Input: part model. Units: mm. Frame: model coordinates. Face numbers are marked on the shaded views. A direction names the side the tool comes from. Give positions to 0.01 mm unless a question says otherwise; leave off trailing zeros. Loops run counter-clockwise (first coordinate to the right, second up) from the corner with the lowest first, then second, coordinate; pieces in that order, holes last. Notation, with made-up numbers: M -3,19 L 43,19 A27 ccw 43,43 Z; hole C 64,27 d5. An arc over 180 degrees is marked long. Answer as a JSON object with one key per item and string values. Group by question number.
1) Section query C-C on y = 0. Return loops of the section in (x, z), plus the area to 3 significant figures.
2) Section query D-D on z = 8.5. Return loops of the section in (x, y), plus the area to 3 significant figures.
3) Section query B-B on x = 0. Return loops of the section in (y, z), plus the area to 3 significant figures.
4) Draft query along X for the marked faces 1, 2, 3 and 4. Return one class per face: +X half, -X half, draft (parallel to the pull), parting line (faces both ways), or undercut.
5) First-contact query: P1, Ø1, axis at x = -7, z = 6, coming from the -Y side; P2, Ø11, axis at x = -3.5, y = 13, coming from the +Z side; P3, Ø3.5, axis at y = 16, z = 27, coming from the -X side; P4, Ø1, axis at x = 18, y = -18, coming from the -Z side. Flat tips, straight axial feed; report the tip coordinate or a pass-through.
6) Section query A-A on z = 15. Return loops of the section in (x, y).
7) Ray query, L1, parallel to Y at x = -15, z = 6; L2, parallel to Y at x = -7, z = 8; L3, parallel to X at y = 17, z = 25.5. Return the intervals inside material, ascending.
8) Access query for the marked faces 5, 6 and 7. Directions: +Z, -Z, +X, -X, +Y, -Y. A direction counts if a zero-diameter tool reaches every point of the face in a straight line with its end or side. Return the directions, or none.
from build123d import *

# Parameters (mm, degrees)
F1_DEPTH    = 5.08
F2_SIZE     = 5.07999
F3_DEPTH    = 12.7
F4_DEPTH    = 12.7
F5_T2_ANGLE = 254.9699407606
F5_T4_ANGLE = 254.9699407606
F8_DEPTH    = 20.32
F9_DEPTH    = 20.32


# Not quite as in the source:
# - a fillet or chamfer that OpenCascade refuses, or shapes differently, is made with other operations: its cross-section is extruded or revolved along the edge and cut away or added
# - a fillet or chamfer is up to 0.001 mm smaller than in the source, because OpenCascade refuses the exact size


with BuildPart() as f1:
    # F0 (on Top) → F1 (new body)
    with BuildSketch(Plane.XY):
        with BuildLine():
            ThreePointArc((34.3164340333, -9.3218), (35.2477374751, -4.7021912858), (35.56, 0))
            ThreePointArc((35.56, 0), (35.2477374751, 4.7021912858), (34.3164340333, 9.3218))
            Line((34.3164340333, 9.3218), (-34.3164340333, 9.3218))
            ThreePointArc((-34.3164340333, 9.3218), (-35.56, 0), (-34.3164340333, -9.3218))
            Line((-34.3164340333, -9.3218), (34.3164340333, -9.3218))
        make_face()
    extrude(amount=F1_DEPTH)

    # F2 (size 5.08 in the source; OpenCascade refuses exactly that, so slightly less here)
    f2_edges = [f1.edges().sort_by_distance(p)[0] for p in [
        (35.56, 0, 5.08),
        (-35.56, 0, 5.08),
    ]]
    chamfer(f2_edges, length=F2_SIZE)

    # F0 (on Top) → F3 (join)
    with BuildSketch(Plane.XY):
        with BuildLine():
            ThreePointArc((-34.3164340333, -9.3218), (0, -35.56), (34.3164340333, -9.3218))
            Line((34.3164340333, -9.3218), (-34.3164340333, -9.3218))
        make_face()
    extrude(amount=F3_DEPTH)

    # F0 (on Top) → F4 (join)
    with BuildSketch(Plane.XY):
        with BuildLine():
            Line((-34.3164340333, 9.3218), (34.3164340333, 9.3218))
            ThreePointArc((34.3164340333, 9.3218), (0, 35.56), (-34.3164340333, 9.3218))
        make_face()
    extrude(amount=F4_DEPTH)

    # F5: chamfer of 12.7 on 2 edges, made by hand

    # F5_s1 → F5_t2 (revolve, cut)
    with BuildSketch(Plane(origin=(0, 0, 0), x_dir=(0, 0, 1), z_dir=(-0.6085532985, -0.7935130011, 0))):
        Polygon((0, -35.56), (12.7, -22.86), (12.7, -35.56), align=None)
    revolve(axis=Axis((0, 0, 12.7), (0, 0, 1)), revolution_arc=F5_T2_ANGLE, mode=Mode.SUBTRACT)

    # F5_s3 → F5_t4 (revolve, cut)
    with BuildSketch(Plane(origin=(0, 0, 0), x_dir=(0, 0, 1), z_dir=(0.6085532985, 0.7935130011, 0))):
        Polygon((0, -35.56), (12.7, -22.86), (12.7, -35.56), align=None)
    revolve(axis=Axis((0, 0, 12.7), (0, 0, 1)), revolution_arc=F5_T4_ANGLE, mode=Mode.SUBTRACT)

    # F6 (on face) → F8 (join)
    with BuildSketch(Plane.XY.offset(12.7)):
        with BuildLine():
            Line((-10.7130363091, -20.1943173452), (-10.7130363091, -9.3218))
            Line((-10.7130363091, -9.3218), (-20.8730363091, -9.3218))
            ThreePointArc((-20.8730363091, -9.3218), (-19.6408996947, -11.6967798638), (-18.1397072045, -13.911528404))
            ThreePointArc((-18.1397072045, -13.911528404), (-14.7644356914, -17.4525367416), (-10.7130363091, -20.1943173452))
        make_face()
        with BuildLine():
            ThreePointArc((10.7130363091, -20.1943173452), (16.7024819777, -15.6079049134), (20.8730363091, -9.3218))
            Line((20.8730363091, -9.3218), (10.7130363091, -9.3218))
            Line((10.7130363091, -9.3218), (10.7130363091, -20.1943173452))
        make_face()
    extrude(amount=F8_DEPTH)

    # F7 (on face) → F9 (join)
    with BuildSketch(Plane.XY.offset(12.7)):
        with BuildLine():
            Line((10.7130363091, 9.3218), (20.8730363091, 9.3218))
            ThreePointArc((20.8730363091, 9.3218), (16.7024819777, 15.6079049134), (10.7130363091, 20.1943173452))
            Line((10.7130363091, 20.1943173452), (10.7130363091, 9.3218))
        make_face()
        with BuildLine():
            Line((-20.8730363091, 9.3218), (-10.7130363091, 9.3218))
            Line((-10.7130363091, 9.3218), (-10.7130363091, 20.1943173452))
            ThreePointArc((-10.7130363091, 20.1943173452), (-16.7024819777, 15.6079049134), (-20.8730363091, 9.3218))
        make_face()
    extrude(amount=F9_DEPTH)


solid = f1.part
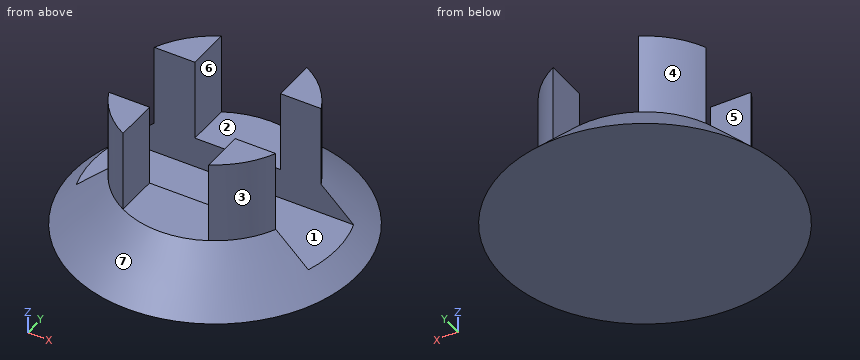
Output:
{
 "1": {"outline": "M -35.56,0 L 35.56,0 L 30.48,5.08 L -30.48,5.08 Z", "area": "335 mm^2"},
 "2": {"outline": "M -25.4,-9.32 A27.06 ccw 25.4,-9.32 Z; M -25.4,9.32 L 25.4,9.32 A27.06 ccw Z", "area": "1,310 mm^2"},
 "3": {"outline": "M -35.56,0 L 35.56,0 L 22.86,12.7 L 9.32,12.7 L 9.32,5.08 L -9.32,5.08 L -9.32,12.7 L -22.86,12.7 Z", "area": "600 mm^2"},
 "4": {"face 1": "draft", "face 2": "undercut", "face 3": "+X half", "face 4": "-X half"},
 "5": {"P1": "stops at y = -29.25", "P2": "stops at z = 12.7", "P3": "stops at x = -17.88", "P4": "stops at z = 0"},
 "6": {"outline": "M -20.87,-9.32 A22.86 ccw -10.71,-20.19 L -10.71,-9.32 Z; M -20.87,9.32 L -10.71,9.32 L -10.71,20.19 A22.86 ccw Z; M 10.71,-20.19 A22.86 ccw 20.87,-9.32 L 10.71,-9.32 Z; M 10.71,9.32 L 20.87,9.32 A22.86 ccw 10.71,20.19 Z"},
 "7": {"L1": "y = -25.47 to -9.32, 9.32 to 25.47", "L2": "y = -26.66 to -9.32, 9.32 to 26.66", "L3": "x = -15.28 to -10.71, 10.71 to 15.28"},
 "8": {"face 5": "+Z, +X, -X", "face 6": "+Z, +Y, -Y", "face 7": "+Z"}
}
